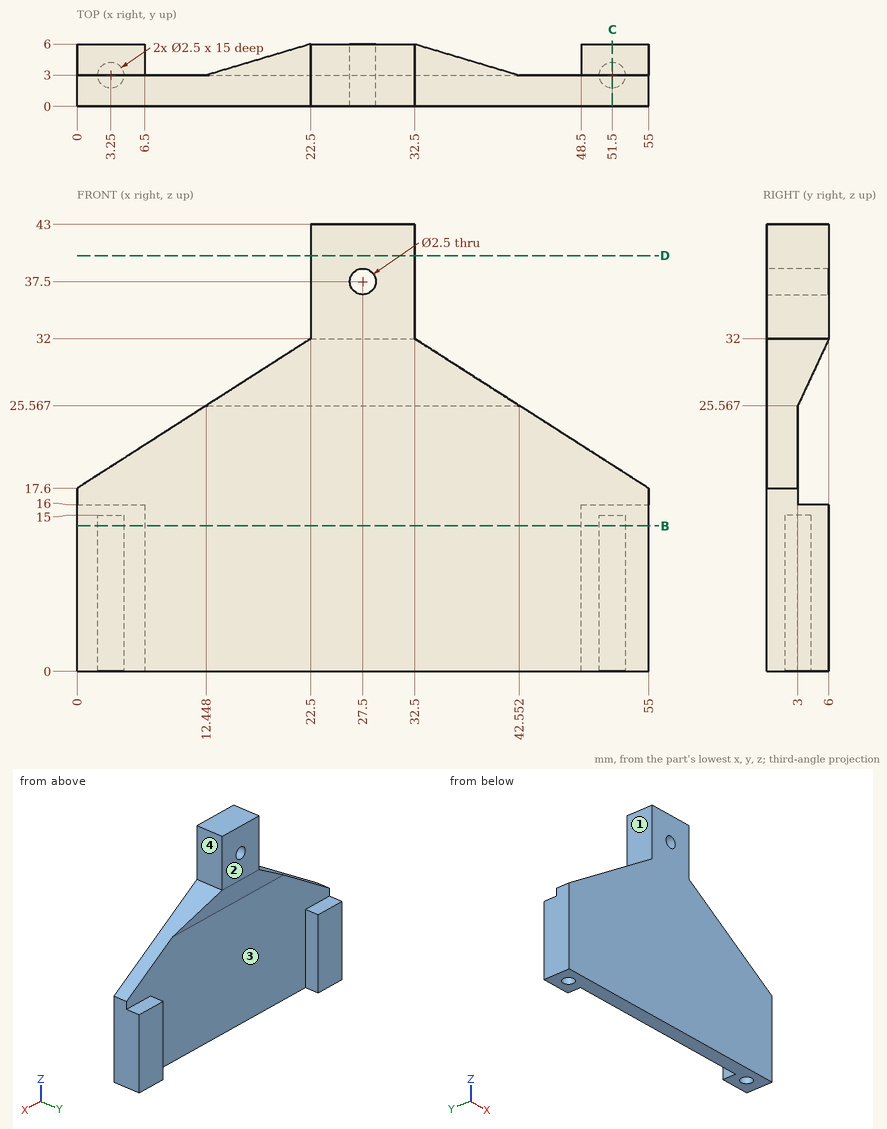
The figure shows three views and two pictorial views of one solid part (mm, origin at its lowest corner). Answer the questions. Coordinates: 2 decimals unless noted, no trailing zeros. Loops run counter-clockwise (first coordinate to the right, second up) from the corner with the lowest first, then second, coordinate; pieces in that order, holes last. Notation, with made-up numbers: M 13,81.25 L 63,81.25 A26 ccw 63,102.25 Z; hole C 28,4.5 d10. An arc over 180 degrees is marked long. Use CSV: the item, a comma, the result in double quotes. Start each with the question number.
(1) Find section C-C, the plane x = 51.5. Give the vertices of the cut face in (y, z).
(2) Consider line 1 (X direction, y = 3.1, z = 7.5) (1 decimal); line 2 (X direction, y = 3.4, z = 37.5); line 3 (X direction, y = 4.45, z = 15). Determine where each line is inside the solid, lowest interval first.
(3) Find section D-D, the plane z = 40. Give the vertices of the cut face in (x, y), then the cut area to 3 significant figures.
(4) For a pull along X with two mould halves and no side action, classify the marked faces 1, 2, 3 and 4 as +X half, -X half, draft (parallel to the pull), parting line (faces both ways), or undercut.
(5) Given pin 1 Ø1.8 at (y, z) = (3.5, 39.5) entering from +X; pin 2 Ø2 at (x, z) = (27.5, 37.5) entering from +Y; pin 3 Ø1.5 at (x, y) = (15.5, 1) entering from +Z; pin 4 Ø13 at (x, z) = (26.5, 7) entering from +Y, each flat-ended and moving along its own axis, determine where each tip first touches the part or whether it passes through.
(6) Find section B-B, the plane z = 14. Give the vertices of the cut face in (x, y), then the cut area to 3 significant figures.
Recorded:
1,outline,"M 0,0 L 1.75,0 L 1.75,15 L 4.25,15 L 4.25,0 L 6,0 L 6,16 L 3,16 L 3,19.84 L 0,19.84 Z"
2,line 1,"x = 0 to 2, 4.5 to 6.5, 48.5 to 50.3, 52.7 to 55"
2,line 2,"x = 22.5 to 26.25, 28.75 to 32.5"
2,line 3,"x = 0 to 6.5, 48.5 to 55"
3,outline,"M 22.5,0 L 32.5,0 L 32.5,6 L 22.5,6 Z"
3,area,"60.0 mm^2"
4,face 1,"-X half"
4,face 2,"draft"
4,face 3,"undercut"
4,face 4,"+X half"
5,pin 1,"stops at x = 32.5"
5,pin 2,"passes through"
5,pin 3,"stops at z = 28"
5,pin 4,"stops at y = 3"
6,outline,"M 0,0 L 55,0 L 55,6 L 48.5,6 L 48.5,3 L 6.5,3 L 6.5,6 L 0,6 Z; hole C 3.25,3 d2.5; hole C 51.5,3 d2.5"
6,area,"194 mm^2"
